CAD build for the part. Positions are in the model's coordinates, mm. A direction names the side the tool comes from. Round coordinates to 2 decimals unless told otherwise and drop trailing zeros. Order: outer loops, then holes, each group sorted by start corner. A loop starts at its lowest first (then second) coordinate and runs counter-clockwise, first axis right, second up. Notation, with made-up numbers: (-7.5, -14) -> (4.5, -14) arc R28 cw to (4.5, 24) -> close; hole circle Ø3 at (43.25, -19). An arc over 180 degrees is marked (long way). Answer as CSV lines item,"result". Start each with the question number.
from build123d import *

# Parameters (mm, degrees)
BOSS_EXTRUDE2_DEPTH     = 24
CUT_EXTRUDE3_DEPTH      = 25
CUT_EXTRUDE3_DEPTH_BACK = 25


with BuildPart() as part:
    # Sketch1<3> → Boss-Extrude2 (new body, symmetric)
    with BuildSketch(Plane.XY):
        Polygon((0, -11), (9.526279442, -5.5), (9.526279442, 5.5), (0, 11), (-9.526279442, 5.5), (-9.526279442, -5.5), align=None)
    extrude(amount=BOSS_EXTRUDE2_DEPTH, both=True)

    # Sketch2 → Cut-Extrude3 (cut, two sides)
    with BuildSketch(Plane.XY) as cut_extrude3_sk:
        Polygon((0, -7.8), (6.75499815, -3.9), (6.75499815, 3.9), (0, 7.8), (-6.75499815, 3.9), (-6.75499815, -3.9), align=None)
    extrude(amount=CUT_EXTRUDE3_DEPTH, mode=Mode.SUBTRACT)
    extrude(cut_extrude3_sk.sketch, amount=-CUT_EXTRUDE3_DEPTH_BACK, mode=Mode.SUBTRACT)


solid = part.part
Item 1: Mould opens along X. For faces 3 (the flat face through (-4.83, -8.21, 0.34)), 4 (the flat face through (4.696, -8.288, 0.336)), 5 (the flat face through (6.755, 0, 0)) say: released by +X, released by -X, zero draft, split by the parting line, or undercut.
Item 2: Pin check, flat tip, straight feed: pin 1 (2 mm diameter, centred on x = -4, y = -3.5, fed in from -Z). Stop position of the tip, or through.
Item 3: Tool access for faces 1 (the flat face through (9.526, 0, 0)), 2 (the flat face through (-6.755, 0, 0)): list every direction of +Z, -Z, +X, -X, +Y, -Y with a clear straight run to the whole face (end or side of a thin tool).
Item 4: Band-saw the part on B-B, the plane z = -17. Give the cut face in (x, y) (3 decimals), and give its area (3 significant figures).
Item 5: Probe line 1 (X direction, y = -2, z = -4) (3 decimals); line 2 (X direction, y = -7, z = 21.5); line 3 (Y direction, x = 0.5, z = 13). List the from-to ranges inside material, lowest first.
Item 6: Band-saw the part on A-A, the plane y = -0.5. Give the cut face in (x, z) (3 decimals), and give its area (3 significant figures).
Item 7: Band-saw the part on C-C, the plane x = 3. Give the cut face in (y, z), and give its area (3 significant figures).
Values:
1,face 3,"released by -X"
1,face 4,"released by +X"
1,face 5,"undercut"
2,pin 1,"through"
3,face 1,"+Z, -Z, +X, +Y, -Y"
3,face 2,"+Z, -Z"
4,outline,"(-9.526, -5.5) -> (0, -11) -> (9.526, -5.5) -> (9.526, 5.5) -> (0, 11) -> (-9.526, 5.5) -> close; hole (-6.755, -3.9) -> (0, -7.8) -> (6.755, -3.9) -> (6.755, 3.9) -> (0, 7.8) -> (-6.755, 3.9) -> close"
4,area,"156 mm²"
5,line 1,"-9.526 to -6.755, 6.755 to 9.526"
5,line 2,"-6.93 to -1.39, 1.39 to 6.93"
5,line 3,"-10.71 to -7.51, 7.51 to 10.71"
6,outline,"(-9.526, -24) -> (-6.755, -24) -> (-6.755, 24) -> (-9.526, 24) -> close; (6.755, -24) -> (9.526, -24) -> (9.526, 24) -> (6.755, 24) -> close"
6,area,"266 mm²"
7,outline,"(-9.27, -24) -> (-6.07, -24) -> (-6.07, 24) -> (-9.27, 24) -> close; (6.07, -24) -> (9.27, -24) -> (9.27, 24) -> (6.07, 24) -> close"
7,area,"307 mm²"
